Can you work these out from the model? Positions are in its coordinate system, mm. A direction names the side the tool comes from. Round coordinates to 2 decimals unless told otherwise and drop trailing zeros. Loops run counter-clockwise (first coordinate to the right, second up) from the corner with the lowest first, then second, coordinate; pieces in that order, holes last. Notation, with made-up numbers: M 42.5,-34.75 L 46.5,-34.75 A14 cw 46.5,-26.75 Z; hole C 58,8 d2. An arc over 180 degrees is marked long. Return JSON: item names as keys, results as strings.
```python
from build123d import *

# Parameters (mm, degrees)
F0_W     = 30
F0_H     = 20
F1_DEPTH = 1.25
F2_W     = 28
F2_H     = 18
F3_DEPTH = 1.8
F4_W     = 26
F4_H     = 16
F5_DEPTH = 1
F6_SIZE  = 5
F7_SIZE  = 5


with BuildPart() as f1:
    # F0 (on Top) → F1 (new body)
    with BuildSketch(Plane.XY):
        Rectangle(F0_W, F0_H)
    extrude(amount=F1_DEPTH)

    # F2 (on face) → F3 (join)
    with BuildSketch(Plane.XY.offset(1.25)):
        Rectangle(F2_W, F2_H)
    extrude(amount=F3_DEPTH)

    # F4 (on face) → F5 (cut)
    with BuildSketch(Plane.XY.offset(3.05)):
        Rectangle(F4_W, F4_H)
    extrude(amount=-F5_DEPTH, mode=Mode.SUBTRACT)

    # F6
    f6_edges = [f1.edges().sort_by_distance(p)[0] for p in [
        (-13, 8, 2.55),
        (13, -8, 2.55),
        (-14, 9, 2.15),
        (14, -9, 2.15),
    ]]
    chamfer(f6_edges, length=F6_SIZE)

    # F7
    f7_edges = [f1.edges().sort_by_distance(p)[0] for p in [
        (15, -10, 0.625),
        (-15, 10, 0.625),
    ]]
    chamfer(f7_edges, length=F7_SIZE)


solid = f1.part
```
Q1. If I drill on line 1 along Y through (x, z) = (-8, 2.7); line 2 along X through (y, z) = (-3, 1.9); line 3 along X through (y, z) = (-7.25, 2.65), over which ranges is the centre line in solid material (lowest first)?
Results:
{"line 1": "y = -9 to -8, 8 to 9", "line 2": "x = -14 to 14", "line 3": "x = -14 to -13, 8.75 to 10.75"}
Q2. Suppose I cut it at A-A, the plane x = -8.5. Please give me the cut outline in (y, z).
Results:
{"outline": "M -10,0 L 10,0 L 10,1.25 L 9,1.25 L 9,3.05 L 7.5,3.05 L 7.5,2.05 L -8,2.05 L -8,3.05 L -9,3.05 L -9,1.25 L -10,1.25 Z"}
Q3. On a 3-axis mill with a long thin cutter (end or side, diameter ignored), from which of +Z, -Z, +X, -X, +Y, -Y can I reach the whole of each face in a straight line? I mean faces 1 (the flat face through (-12, 6, 2)), 2 (the flat face through (2, 9, 2)), 3 (the flat face through (12, -6, 2)), 4 (the flat face through (-14, -3, 2)), 5 (the flat face through (13, 2.4, 2.6)). Say none if no direction works.
Results:
{"face 1": "+Z, -X, +Y", "face 2": "+Z, +X, -X, +Y", "face 3": "+Z, +X, -Y", "face 4": "+Z, -X, +Y, -Y", "face 5": "+Z"}
Q4. I'm going to push flat-ended pins straight in: pin 1 Ø0.8 at (y, z) = (4, 2.5) entering from -X; pin 2 Ø8 at (x, y) = (5.5, 2.5) entering from +Z; pin 3 Ø0.5 at (x, z) = (4.5, 2.5) entering from -Y. Where does each tip first touch, or does it pass through?
Results:
{"pin 1": "stops at x = -14", "pin 2": "stops at z = 2.05", "pin 3": "stops at y = -9"}
Q5. Suppose I cut it at B-B, the plane y = 1. Please give me the cut outline in (x, z).
Results:
{"outline": "M -15,0 L 15,0 L 15,1.25 L 14,1.25 L 14,3.05 L 13,3.05 L 13,2.05 L -13,2.05 L -13,3.05 L -14,3.05 L -14,1.25 L -15,1.25 Z"}
Q6. Thinking about a two-plate mould opening in Y: for faces 6 (the flat face through (-3, -9, 2)), 7 (the flat face through (-0.1, -9.6, 1.25)), 8 (the flat face through (0, 0, 2.05)), which applies, pulls with the +Y half, pulls with the -Y half, needs draft (parallel to the pull), parting line crosses it, or undercut?
Results:
{"face 6": "pulls with the -Y half", "face 7": "needs draft", "face 8": "undercut"}
Q7. Suppose I cut it at C-C, the plane z = 0.6. Please give me the cut outline in (x, y), plus the area to 3 significant figures.
Results:
{"outline": "M -15,-10 L 10,-10 L 15,-5 L 15,10 L -10,10 L -15,5 Z", "area": "575 mm2"}
